Geometry check sheet. Reference: the model listing, model coordinates, mm. Give positions to 0.01 mm unless a question says otherwise; leave off trailing zeros. Write each loop counter-clockwise with the first axis right and the second up, starting at its lowest first coordinate (ties: lowest second). Pieces come first, ordered by that corner, then holes. Notation, with made-up numbers: (-0.75, -31) - (58.25, -31) arc R20 cw to (58.25, 7) - close; hole circle Ø8 at (18, 41). An arc over 180 degrees is marked (long way). Use a Markdown table: item, result.
```python
from build123d import *

# Parameters (mm, degrees)
BOSS_EXTRUDE1_DEPTH = 3.175
CUT_EXTRUDE1_DEPTH  = 4.175


with BuildPart() as part:
    # Sketch1 → Boss-Extrude1 (new body)
    with BuildSketch(Plane(origin=(0, 0, 0), x_dir=(1, 0, 0), z_dir=(0, 1, 0))):
        Polygon((0, 0), (76.2, 0), (76.2, 12.7), (78.6892, 12.7), (78.6892, 25.4), (76.2, 25.4), (76.2, 38.1), (78.6892, 38.1), (78.6892, 50.8), (76.2, 50.8), (76.2, 63.5), (78.6892, 63.5), (78.6892, 76.2), (76.2, 76.2), (76.2, 88.9), (78.6892, 88.9), (78.6892, 101.6), (-2.4892, 101.6), (-2.4892, 88.9), (0, 88.9), (0, 76.2), (-2.4892, 76.2), (-2.4892, 63.5), (0, 63.5), (0, 50.8), (-2.4892, 50.8), (-2.4892, 38.1), (0, 38.1), (0, 25.4), (-2.4892, 25.4), (-2.4892, 12.7), (0, 12.7), align=None)
    extrude(amount=BOSS_EXTRUDE1_DEPTH)

    # Sketch2 → Cut-Extrude1 (cut, through all)
    with BuildSketch(Plane(origin=(0, 3.175, 0), x_dir=(1, 0, 0), z_dir=(0, 1, 0))):
        Polygon((78.6892, 101.6), (78.5622, 101.6), (78.5622, 89.027), (76.073, 89.027), (76.073, 76.073), (78.5622, 76.073), (78.5622, 63.627), (76.073, 63.627), (76.073, 50.673), (78.5622, 50.673), (78.5622, 38.227), (76.073, 38.227), (76.073, 25.273), (78.5622, 25.273), (78.5622, 12.827), (76.073, 12.827), (76.073, 0), (76.2, 0), (76.2, 12.7), (78.6892, 12.7), (78.6892, 25.4), (76.2, 25.4), (76.2, 38.1), (78.6892, 38.1), (78.6892, 50.8), (76.2, 50.8), (76.2, 63.5), (78.6892, 63.5), (78.6892, 76.2), (76.2, 76.2), (76.2, 88.9), (78.6892, 88.9), align=None)
        Polygon((-2.3622, 101.6), (-2.4892, 101.6), (-2.4892, 88.9), (0, 88.9), (0, 76.2), (-2.4892, 76.2), (-2.4892, 63.5), (0, 63.5), (0, 50.8), (-2.4892, 50.8), (-2.4892, 38.1), (0, 38.1), (0, 25.4), (-2.4892, 25.4), (-2.4892, 12.7), (0, 12.7), (0, 0), (0.127, 0), (0.127, 12.827), (-2.3622, 12.827), (-2.3622, 25.273), (0.127, 25.273), (0.127, 38.227), (-2.3622, 38.227), (-2.3622, 50.673), (0.127, 50.673), (0.127, 63.627), (-2.3622, 63.627), (-2.3622, 76.073), (0.127, 76.073), (0.127, 89.027), (-2.3622, 89.027), align=None)
    extrude(amount=-CUT_EXTRUDE1_DEPTH, mode=Mode.SUBTRACT)


solid = part.part
```
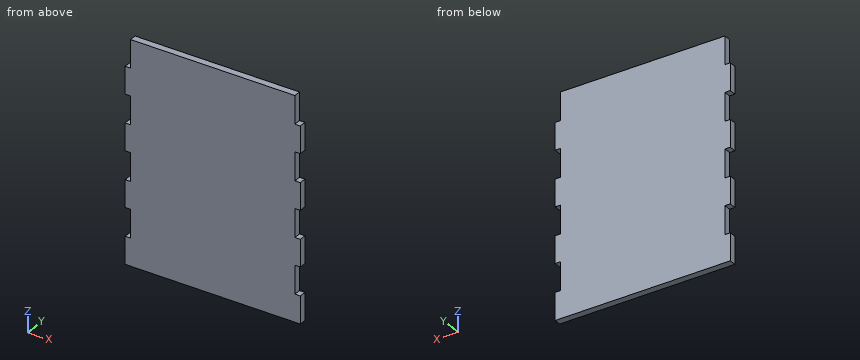
1) Depth check by flat-ended pin: P1, Ø1.2, axis at x = 77, y = 1, coming from the +Z side; P2, Ø1.6, axis at y = 2.5, z = -30, coming from the -X side; P3, Ø10, axis at x = 60.5, z = -29.5, coming from the -Y side. Enter the tip coordinate at first touch or a pass-through.
Working result:
| item | result |
|---|---|
| P1 | stops at z = -12.83 |
| P2 | stops at x = 0.13 |
| P3 | stops at y = 0 |
2) Section check B-B on z = -11. Record the boundary of the cut face in (x, y) (3 decimals), then the cut area to 3 significant figures.
Working result:
| item | result |
|---|---|
| outline | (0.127, 0) - (76.073, 0) - (76.073, 3.175) - (0.127, 3.175) - close |
| area | 241 mm² |
3) Material ranges on L1, parallel to X at y = 0.95, z = -29, recorded low to high. Write a range as from..to.
Working result:
| item | result |
|---|---|
| L1 | x = 0.13..76.07 |
